```python
from build123d import *

# Parameters (mm, degrees)
SKETCH2_W            = 150
SKETCH2_H            = 150
BOSS_EXTRUDE1_DEPTH  = 1
SKETCH4_R            = 0.79375
CUT_EXTRUDE1_DEPTH   = 160.418359102
LPATTERN1_COUNT      = 5
LPATTERN1_PITCH      = 27
LPATTERN1_COUNT_DIR2 = 6
LPATTERN1_PITCH_DIR2 = 22
M3_CLEARANCE_HOLE1_D = 3.4
SKETCH8_R            = 1.5
CUT_EXTRUDE2_DEPTH   = 160.418359102


with BuildPart() as part:
    # Sketch2 → Boss-Extrude1 (new body)
    with BuildSketch(Plane(origin=(0, 0, 0), x_dir=(0, 0, -1), z_dir=(1, 0, 0))):
        with Locations((34.101040119, -41.233283804)):
            Rectangle(SKETCH2_W, SKETCH2_H)
    extrude(amount=BOSS_EXTRUDE1_DEPTH)

    # Sketch4 → Cut-Extrude1 (cut, through all)
    with BuildSketch(Plane(origin=(1, 0, 0), x_dir=(0, 0, -1), z_dir=(1, 0, 0))):
        with Locations((-22.398959881, 11.548854602)):
            Circle(SKETCH4_R)
        with Locations((-17.398959881, 11.548854602)):
            Circle(SKETCH4_R)
        with Locations((-12.398959881, 11.548854602)):
            Circle(SKETCH4_R)
    cut_extrude1 = extrude(amount=-CUT_EXTRUDE1_DEPTH, mode=Mode.SUBTRACT)

    # LPattern1: Cut-Extrude1 5 × 6
    with Locations(*[(0, -j * LPATTERN1_PITCH_DIR2, -i * LPATTERN1_PITCH) for i in range(LPATTERN1_COUNT) for j in range(LPATTERN1_COUNT_DIR2) if (i, j) != (0, 0)]):
        add(cut_extrude1, mode=Mode.SUBTRACT)

    # M3 Clearance Hole1 (through all)
    with Locations(Plane(origin=(1, 0, 0), x_dir=(0, 0, -1), z_dir=(1, 0, 0))):
        with Locations((-36.898959881, 29.766716196), (105.101040119, 29.766716196), (105.101040119, -112.233283804), (-36.898959881, -112.233283804)):
            Hole(M3_CLEARANCE_HOLE1_D / 2)

    # Sketch8 → Cut-Extrude2 (cut, through all)
    with BuildSketch(Plane(origin=(1, 0, 0), x_dir=(0, 0, -1), z_dir=(1, 0, 0))):
        with Locations((39.101040119, 29.766716196)):
            Circle(SKETCH8_R)
        with Locations((-36.898959881, -16.233283804)):
            Circle(SKETCH8_R)
        with Locations((9.101040119, -112.233283804)):
            Circle(SKETCH8_R)
        with Locations((105.101040119, -66.233283804)):
            Circle(SKETCH8_R)
    extrude(amount=-CUT_EXTRUDE2_DEPTH, mode=Mode.SUBTRACT)


solid = part.part
```
Input: part model. Units: mm. Frame: model coordinates. Round coordinates to 2 decimals unless told otherwise and drop trailing zeros. Answer as CSV lines item,"result".
1. Mould query, pull axis Z, two halves, no side actions, for faces 1 (the flat face through (0, -40, -33)), 2 (the cylindrical face through (0.5, 29.8, 35.2)). Classes: +Z half, -Z half, draft (parallel to the pull), parting line (faces both ways), or undercut.
Geometry says:
face 1,"draft"
face 2,"undercut"
2. Ray query, L1, parallel to Y at x = 0.15, z = -40; L2, parallel to Y at x = 0.3, z = -38. Return the intervals inside material, ascending. Write a range as [from, to].
Geometry says:
L1,"y = [-116.23, 28.57], [30.97, 33.77]"
L2,"y = [-116.23, 28.75], [30.79, 33.77]"
3. Contact query for a flat-ended pin moving along its axis: P1, Ø1.3, axis at y = -54.45, z = -31.6, coming from the -X side. Output: stop coordinate, or through.
Geometry says:
P1,"passes through"
